```python
from build123d import *

# Parameters (mm, degrees)
SKETCH1_W           = 41.91
SKETCH1_H           = 41.91
SKETCH1_R           = 12.7
SKETCH1_R_2         = 1.714924581
BOSS_EXTRUDE1_DEPTH = 3.81
SKETCH2_W           = 48.006
SKETCH2_H           = 41.91
BOSS_EXTRUDE2_DEPTH = 3.81
LOFT1_START         = -20.955
LOFT1_DEPTH         = 41.91


# Read off the part's stored shape, not the designer's step: Loft1
with BuildPart() as part:
    # Sketch1 → Boss-Extrude1 (new body)
    with BuildSketch(Plane(origin=(0, 0, 0), x_dir=(0, 0, -1), z_dir=(1, 0, 0))):
        Rectangle(SKETCH1_W, SKETCH1_H)
        with Locations(Location((0, 0, 0), (0, 0, 180))):
            Circle(SKETCH1_R, mode=Mode.SUBTRACT)
        with Locations(Location((14.112032399, 14.112032399, 0), (0, 0, 180))):
            Circle(SKETCH1_R_2, mode=Mode.SUBTRACT)
        with Locations(Location((-14.112032399, -14.112032399, 0), (0, 0, 180))):
            Circle(SKETCH1_R_2, mode=Mode.SUBTRACT)
        with Locations(Location((-14.112032399, 14.112032399, 0), (0, 0, 180))):
            Circle(SKETCH1_R_2, mode=Mode.SUBTRACT)
        with Locations(Location((14.112032399, -14.112032399, 0), (0, 0, 180))):
            Circle(SKETCH1_R_2, mode=Mode.SUBTRACT)
    extrude(amount=BOSS_EXTRUDE1_DEPTH)



with BuildPart() as body_2:
    # Sketch2 → Boss-Extrude2 (new body)
    with BuildSketch(Plane(origin=(0, 0, -20.955), x_dir=(-1, 0, 0), z_dir=(0, 0, -1))):
        with Locations((24.003, 0)):
            Rectangle(SKETCH2_W, SKETCH2_H)
        with BuildLine():
            Line((10.094228129, 7.189050974), (28.005771871, 7.189050974))
            ThreePointArc((28.005771871, 7.189050974), (30.545771871, 9.729050974), (28.005771871, 12.269050974))
            Line((28.005771871, 12.269050974), (10.094228129, 12.269050974))
            ThreePointArc((10.094228129, 12.269050974), (7.554228129, 9.729050974), (10.094228129, 7.189050974))
        make_face(mode=Mode.SUBTRACT)
        with BuildLine():
            Line((10.094228129, -7.189050974), (28.005771871, -7.189050974))
            ThreePointArc((28.005771871, -7.189050974), (30.545771871, -9.729050974), (28.005771871, -12.269050974))
            Line((28.005771871, -12.269050974), (10.094228129, -12.269050974))
            ThreePointArc((10.094228129, -12.269050974), (7.554228129, -9.729050974), (10.094228129, -7.189050974))
        make_face(mode=Mode.SUBTRACT)
    extrude(amount=BOSS_EXTRUDE2_DEPTH)


with BuildPart() as part_1:
    add(part.part)

    add(body_2.part)  # Loft1 merges body 2
    # Loft1 outline → Loft1 (add)
    with BuildSketch(Plane(origin=(0, 0, 0), x_dir=(1, 0, 0), z_dir=(0, 1, 0)).offset(LOFT1_START)):
        Polygon((3.81, 20.955), (0, 24.765), (0, 20.955), align=None)
    extrude(amount=LOFT1_DEPTH)


solid = part_1.part
```
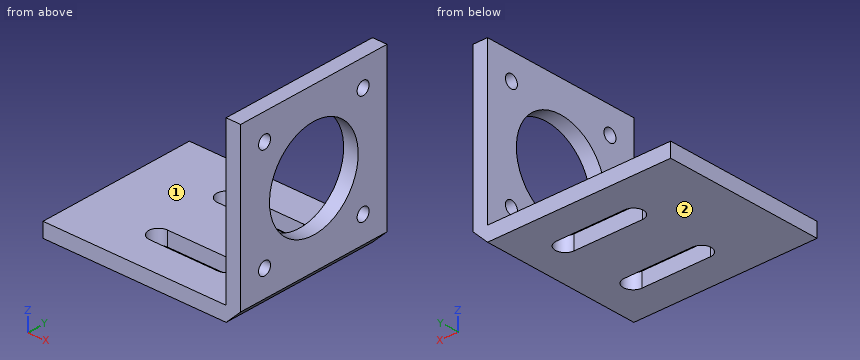
Could you check a few things on this model? Use its own coordinates, in mm. Face numbers are marked on the shaded views. A direction names the side the tool comes from. Round coordinates to 2 decimals unless told otherwise and drop trailing zeros. Write each loop counter-clockwise with the first axis right and the second up, starting at its lowest first coordinate (ties: lowest second). Pieces come first, ordered by that corner, then holes. Notation, with made-up numbers: M -34,-25.75 L -1,-25.75 A17 cw -1,-6.75 Z; hole C 54.5,44.25 d8. An arc over 180 degrees is marked long. Answer in a Markdown table with one row per item. Add a question column.
Q1. Will these pins go through, and if not, where does the flat tip stop? pin 1 Ø8 at (y, z) = (-11.5, 0.5) entering from -X; pin 2 Ø8 at (x, y) = (-21.5, 0) entering from +Z (3 decimals).
Q2. Imagine slicing it at C-C (y = 15). Please give me the cut outline in (x, z) (3 decimals), then the cut area to 3 significant figures.
Q3. If I drill on line 1 (Y direction, x = 2.8, z = 0) (3 decimals); line 2 (X direction, y = -6, z = 16); line 3 (Z direction, x = -26.5, y = -15) (3 decimals), over which ranges is the centre line in solid material (lowest first)? Write a range as from..to.
Q4. On a 3-axis mill with a long thin cutter (end or side, diameter ignored), from which of +Z, -Z, +X, -X, +Y, -Y can I reach the whole of each face in a straight line? I mean the marked faces 1 and 2. Say none if no direction works.
Q5. Imagine slicing it at D-D (z = 5). Please give me the cut outline in (x, y) (3 decimals).
Q6. Imagine slicing it at B-B (z = 0). Please give me the cut outline in (x, y) (3 decimals), then the cut area to 3 significant figures.
Q7. Imagine slicing it at A-A (y = 0). Please give me the cut outline in (x, z) (3 decimals), then the cut area to 3 significant figures.
Values:
| question | item | result |
|---|---|---|
| 1 | pin 1 | x = 0 |
| 1 | pin 2 | z = -20.955 |
| 2 | outline | M -48.006,-24.765 L 0,-24.765 L 3.81,-20.955 L 3.81,-15.579 L 0,-15.579 L 0,-20.955 L -48.006,-20.955 Z; M 0,-12.645 L 3.81,-12.645 L 3.81,12.645 L 0,12.645 Z; M 0,15.579 L 3.81,15.579 L 3.81,20.955 L 0,20.955 Z |
| 2 | area | 327 mm^2 |
| 3 | line 1 | -20.955..-12.7, 12.7..20.955 |
| 3 | line 2 | 0..3.81 |
| 3 | line 3 | -24.765..-20.955 |
| 4 | face 1 | +Z, -X, +Y, -Y |
| 4 | face 2 | -Z, +X, -X, +Y, -Y |
| 5 | outline | M 0,-20.955 L 3.81,-20.955 L 3.81,-11.674 L 0,-11.674 Z; M 0,11.674 L 3.81,11.674 L 3.81,20.955 L 0,20.955 Z |
| 6 | outline | M 0,-20.955 L 3.81,-20.955 L 3.81,-12.7 L 0,-12.7 Z; M 0,12.7 L 3.81,12.7 L 3.81,20.955 L 0,20.955 Z |
| 6 | area | 62.9 mm^2 |
| 7 | outline | M -48.006,-24.765 L 0,-24.765 L 3.81,-20.955 L 3.81,-12.7 L 0,-12.7 L 0,-20.955 L -48.006,-20.955 Z; M 0,12.7 L 3.81,12.7 L 3.81,20.955 L 0,20.955 Z |
| 7 | area | 253 mm^2 |
